```python
from build123d import *

# Parameters (mm, degrees)
F1_DEPTH = 5
F2_R     = 4
F3_DEPTH = 10


with BuildPart() as f1:
    # F0 (on Right) → F1 (new body)
    with BuildSketch(Plane.YZ):
        with BuildLine():
            Line((9, 9), (19, 9))
            Line((19, 9), (19, 11))
            Line((19, 11), (9, 11))
            ThreePointArc((9, 11), (1.221825, 7.778175), (-2, 0))
            Line((-2, 0), (-2, -17))
            ThreePointArc((-2, -17), (2.129794, -26.970206), (12.1, -31.1))
            Line((12.1, -31.1), (20.1, -31.1))
            Line((20.1, -31.1), (20.1, -29.1))
            Line((20.1, -29.1), (12.1, -29.1))
            ThreePointArc((12.1, -29.1), (3.544008, -25.555992), (0, -17))
            Line((0, -17), (0, 0))
            ThreePointArc((0, 0), (2.636039, 6.363961), (9, 9))
        make_face()
    extrude(amount=F1_DEPTH)

    # F2 (on face) → F3 (cut)
    with BuildSketch(Plane(origin=(0, 0, -31.1), x_dir=(1, 0, 0), z_dir=(0, 0, -1))):
        with Locations((7.078093, -7.6)):
            Circle(F2_R)
    extrude(amount=-F3_DEPTH, mode=Mode.SUBTRACT)


solid = f1.part
```
Work out the finished part from the listing and answer in its coordinate system (mm). A direction names the side the tool comes from. Give positions to 0.01 mm unless a question says otherwise; leave off trailing zeros. Order: outer loops, then holes, each group sorted by start corner. A loop starts at its lowest first (then second) coordinate and runs counter-clockwise, first axis right, second up.
1. Section D-D, the plane z = -11 is taken. Determine the outline of the cut face in (x, y), and give its area (3 significant figures).
Result sheet:
outline: (0, -2) - (5, -2) - (5, 0) - (0, 0) - close
area: 10.0 mm2
2. Section B-B, the plane x = 4.15 is taken. Determine the outline of the cut face in (y, z), and give its area (3 significant figures).
Result sheet:
outline: (-2, -17) arc R14.1 ccw to (4.87, -29.11) - (4.87, -26.71) arc R12.1 cw to (0, -17) - (0, 0) arc R9 cw to (9, 9) - (19, 9) - (19, 11) - (9, 11) arc R11 ccw to (-2, 0) - close; (10.33, -30.99) arc R14.1 ccw to (12.1, -31.1) - (20.1, -31.1) - (20.1, -29.1) - (12.1, -29.1) arc R12.1 cw to (10.33, -28.97) - close
area: 131 mm2
3. Each of these flat-tipped pins is pushed along its axis until it touches: P1, Ø3, axis at x = 2.5, z = -1.5, coming from the +Y side; P2, Ø1.5, axis at x = 4, y = 7, coming from the -Z side; P3, Ø1, axis at x = 1.5, z = 9.5, coming from the +Y side. Where does it stop, or does it pass through?
Result sheet:
P1: stops at y = 0
P2: stops at z = 8.57
P3: stops at y = 19
4. Straight lines are drawn through the part: L1, parallel to Z at x = 2.8, y = 12.25; L2, parallel to Y at x = 3.4, z = -6; L3, parallel to Z at x = 4.1, y = 10. For each, find the intervals that lie inside material, in ascending order.
Result sheet:
L1: z = -31.1 to -29.1, 9 to 11
L2: y = -2 to 0
L3: z = 9 to 11
5. Section C-C, the plane x = 1.05 is taken. Determine the outline of the cut face in (y, z).
Result sheet:
outline: (-2, -17) arc R14.1 ccw to (12.1, -31.1) - (20.1, -31.1) - (20.1, -29.1) - (12.1, -29.1) arc R12.1 cw to (0, -17) - (0, 0) arc R9 cw to (9, 9) - (19, 9) - (19, 11) - (9, 11) arc R11 ccw to (-2, 0) - close
6. Section A-A, the plane y = 18.25 is taken. Determine the outline of the cut face in (x, z).
Result sheet:
outline: (0, -31.1) - (5, -31.1) - (5, -29.1) - (0, -29.1) - close; (0, 9) - (5, 9) - (5, 11) - (0, 11) - close
7. For faces 1 (the cylindrical face through (3.08, 7.54, -29.18)), 2 (the cylindrical face through (2.46, 3.64, -25.65)), 3 (the flat face through (2, 19, 10)), determine the directions among +Z, -Z, +X, -X, +Y, -Y from which every point of the face is accessible in a straight line to the end or side of a thin tool.
Result sheet:
face 1: -Z, +X
face 2: +X, -X, +Y
face 3: +Z, +X, -X, +Y
8. The mould has two halves that part along Z. Classify faces 4 (the flat face through (2, 14, 11)), 5 (the flat face through (5, 15, -30)), 6 (the cylindrical face through (2.465, 2.566, 6.294)): released by +Z, released by -Z, zero draft, split by the parting line, or undercut.
Result sheet:
face 4: released by +Z
face 5: zero draft
face 6: undercut
